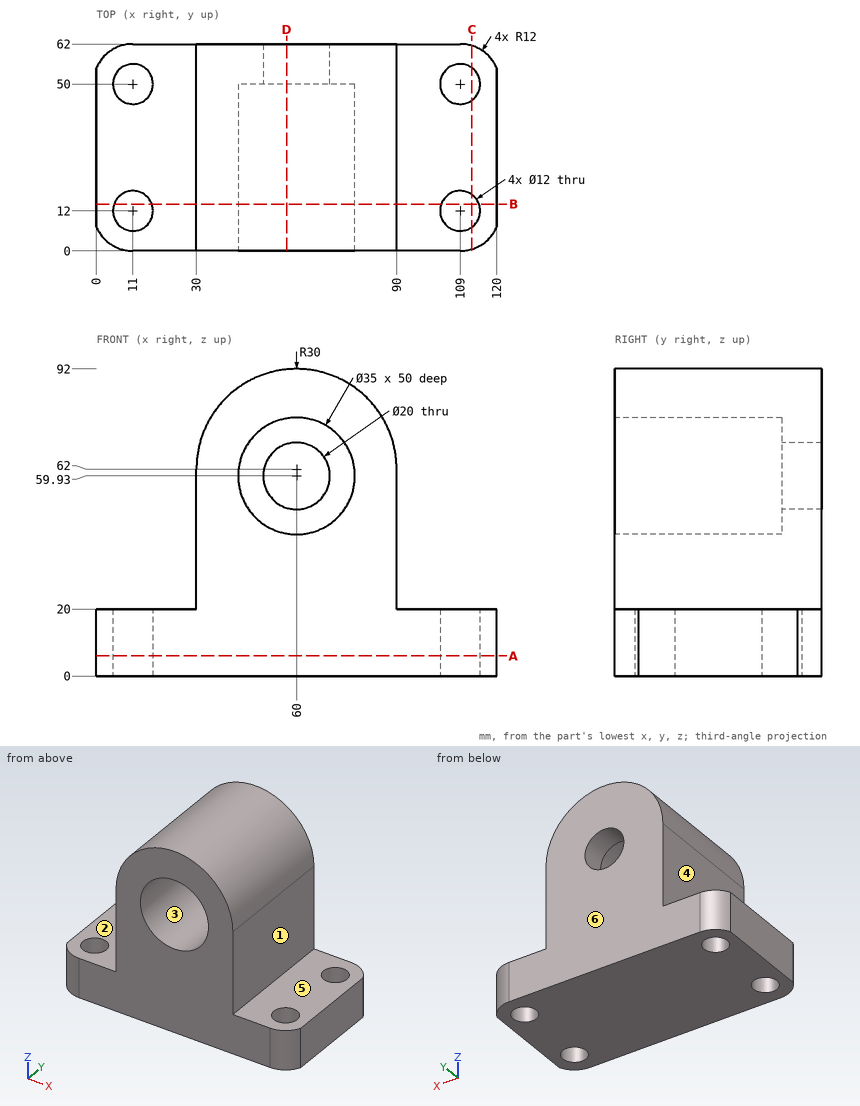
Design review of the part shown in the three views and the two pictorial views. Dimensions are in mm from the part's minimum x, y and z. A direction names the side the tool comes from. Give positions to 0.01 mm unless a question says otherwise; leave off trailing zeros. Loops run counter-clockwise (first coordinate to the right, second up) from the corner with the lowest first, then second, coordinate; pieces in that order, holes last. Notation, with made-up numbers: M -2,-32.5 L 29,-32.5 A11 ccw 29,-20.5 Z; hole C 87.25,54.25 d5. An arc over 180 degrees is marked long. Answer as a JSON object with one key per item and string values. Group by question number.
Q1. Add section B-B on y = 14. Give the boundary of the cut face in (x, z).
Q2. For probe 1 along Y at (x, z) = (11, 9.75); probe 2 along Z at (x, y) = (60, 14.5); probe 3 along Z at (x, y) = (60, 53), list the stretches that pass through material, from the lowest coordinate up. Write a range as [from, to].
Q3. Add section A-A on z = 6. Give the boundary of the cut face in (x, y), and give its area (3 significant figures).
Q4. Add section C-C on x = 112.5. Give the boundary of the cut face in (y, z), and give its area (3 significant figures).
Q5. Add section D-D on x = 57. Give the boundary of the cut face in (y, z).
Q6. Mouldability with a two-part tool opening along X and no side actions: class the marked faces 1, 2 and 3 as +X half, -X half, draft (parallel to the pull), parting line (faces both ways), or undercut.
Q7. Tool access review of the marked faces 4, 5 and 6: name each direction out of +Z, -Z, +X, -X, +Y, -Y from which nothing blocks a thin tool from reaching the whole face with its end or side.
Q8. Insertion check: P1, Ø1, axis at y = 17.5, z = 31, coming from the -X side; P2, Ø15.5, axis at x = 109, y = 12, coming from the +Z side; P3, Ø5, axis at y = 18, z = 29.5, coming from the +X side. Each pin has a flat end and moves straight along its axis. Give the tip position at first contact, or say it passes through.
Checked values:
{
 "1": {"outline": "M 0,0 L 5.34,0 L 5.34,20 L 0,20 Z; M 16.66,0 L 103.34,0 L 103.34,20 L 90,20 L 90,62 A30 ccw 30,62 L 30,20 L 16.66,20 Z; M 114.66,0 L 120,0 L 120,20 L 114.66,20 Z; hole C 60,59.93 d35"},
 "2": {"probe 1": "[0, 6], [18, 44], [56, 62]", "probe 2": "[0, 42.43], [77.43, 92]", "probe 3": "[0, 49.93], [69.93, 92]"},
 "3": {"outline": "M 0,7.2 A12 ccw 11,0 L 109,0 A12 ccw 120,7.2 L 120,54.8 A12 ccw 109,62 L 11,62 A12 ccw 0,54.8 Z; hole C 11,12 d12; hole C 11,50 d12; hole C 109,12 d12; hole C 109,50 d12", "area": "6,900 mm²"},
 "4": {"outline": "M 0.52,0 L 7.13,0 L 7.13,20 L 0.52,20 Z; M 16.87,0 L 45.13,0 L 45.13,20 L 16.87,20 Z; M 54.87,0 L 61.48,0 L 61.48,20 L 54.87,20 Z", "area": "829 mm²"},
 "5": {"outline": "M 0,0 L 62,0 L 62,50.39 L 50,50.39 L 50,42.69 L 0,42.69 Z; M 0,77.17 L 50,77.17 L 50,69.47 L 62,69.47 L 62,91.85 L 0,91.85 Z"},
 "6": {"face 1": "+X half", "face 2": "draft", "face 3": "undercut"},
 "7": {"face 4": "+Z, -X, +Y, -Y", "face 5": "+Z, +X, +Y, -Y", "face 6": "+Z, -Z, +X, -X, +Y"},
 "8": {"P1": "x = 30", "P2": "z = 20", "P3": "x = 90"}
}
